Can you work these out from the model? Positions are in its coordinate system, mm. A direction names the side the tool comes from. Give positions to 0.01 mm unless a question says otherwise; leave off trailing zeros. Loops run counter-clockwise (first coordinate to the right, second up) from the corner with the lowest first, then second, coordinate; pieces in that order, holes last. Notation, with made-up numbers: (77, 85) - (131, 85) arc R13 cw to (131, 97) - close; hole circle Ø7 at (44.25, -14.5). An arc over 180 degrees is marked (long way). Answer as a JSON object with one key per item and string values.
```python
from build123d import *

# Parameters (mm, degrees)
SKETCH_1_W          = 68
SKETCH_1_H          = 65
EXTRUDE_1_DEPTH     = 68
SKETCH_2_W          = 65
SKETCH_2_H          = 65
CUT_EXTRUDE_1_DEPTH = 65
FILLET_1_R          = 1
SKETCH_6_R          = 2.6
SKETCH_6_R_2        = 19.1
CUT_EXTRUDE_4_DEPTH = 51
CUT_EXTRUDE_5_DEPTH = 51


with BuildPart() as part:
    # 草图1 → 凸台-拉伸1 (new body)
    with BuildSketch(Plane(origin=(0, 0, 0), x_dir=(0, 0, -1), z_dir=(1, 0, 0))):
        Rectangle(SKETCH_1_W, SKETCH_1_H)
    extrude(amount=EXTRUDE_1_DEPTH)

    # 草图2 → 切除-拉伸1 (cut)
    with BuildSketch(Plane(origin=(68, 0, 0), x_dir=(0, 0, -1), z_dir=(1, 0, 0))):
        with Locations((1.5, 0)):
            Rectangle(SKETCH_2_W, SKETCH_2_H)
    extrude(amount=-CUT_EXTRUDE_1_DEPTH, mode=Mode.SUBTRACT)

    # 圆角1
    fillet_1_edges = [part.edges().sort_by_distance(p)[0] for p in [
        (0, 0, 34),
    ]]
    fillet(fillet_1_edges, radius=FILLET_1_R)

    # 草图6 → 切除-拉伸4 (cut)
    with BuildSketch(Plane(origin=(0, 0, 31), x_dir=(-1, 0, 0), z_dir=(0, 0, -1))):
        with Locations((-62.5, 23.5)):
            Circle(SKETCH_6_R)
        with Locations((-15.5, 23.5)):
            Circle(SKETCH_6_R)
        with Locations((-39, 0)):
            Circle(SKETCH_6_R_2)
        with Locations((-15.5, -23.5)):
            Circle(SKETCH_6_R)
        with Locations((-62.5, -23.5)):
            Circle(SKETCH_6_R)
        Polygon((-68, 32.5), (-68, 27), (-62.5, 32.5), align=None)
        Polygon((-68, -27), (-62.5, -32.5), (-68, -32.5), align=None)
    extrude(amount=-CUT_EXTRUDE_4_DEPTH, mode=Mode.SUBTRACT)

    # 草图7 → 切除-拉伸5 (cut)
    with BuildSketch(Plane(origin=(3, 0, 0), x_dir=(0, 0, -1), z_dir=(1, 0, 0))):
        Polygon((28.5, 32.5), (34, 32.5), (34, 27), align=None)
        with BuildLine():
            Line((-18, 22.1), (24, 22.1))
            ThreePointArc((24, 22.1), (26.1, 20), (24, 17.9))
            Line((24, 17.9), (-18, 17.9))
            ThreePointArc((-18, 17.9), (-20.1, 20), (-18, 22.1))
        make_face()
        Polygon((34, -32.5), (34, -27), (28.5, -32.5), align=None)
        with BuildLine():
            Line((-18, -17.9), (24, -17.9))
            ThreePointArc((24, -17.9), (26.1, -20), (24, -22.1))
            Line((24, -22.1), (-18, -22.1))
            ThreePointArc((-18, -22.1), (-20.1, -20), (-18, -17.9))
        make_face()
    extrude(amount=-CUT_EXTRUDE_5_DEPTH, mode=Mode.SUBTRACT)


solid = part.part
```
1) Imagine slicing it at B-B on z = -18. Write out the boundary of the cut face in (x, y).
Check sheet entries:
{"outline": "(0, -32.5) - (3, -32.5) - (3, -22.1) - (0, -22.1) - close; (0, -17.9) - (3, -17.9) - (3, 17.9) - (0, 17.9) - close; (0, 22.1) - (3, 22.1) - (3, 32.5) - (0, 32.5) - close"}
2) Imagine slicing it at A-A on y = 23.5. Write out the boundary of the cut face in (x, z).
Check sheet entries:
{"outline": "(0, -34) - (3, -34) - (3, 31) - (12.9, 31) - (12.9, 34) - (1, 34) arc R1 ccw to (0, 33) - close; (18.1, 31) - (59.9, 31) - (59.9, 34) - (18.1, 34) - close; (65.1, 31) - (68, 31) - (68, 34) - (65.1, 34) - close"}
3) Which directions (+Z, -Z, +X, -X, +Y, -Y) give clear straight access to the entire face, cutting with the end or side of a thin tool? Please do faces 1 (the flat face through (65, 30, 32)), 2 (the cylindrical face through (1.5, 20, -26.1)), 3 (the flat face through (22, -15, 31)).
Check sheet entries:
{"face 1": "+Z, -Z, +X, +Y", "face 2": "+X, -X", "face 3": "-Z, +X, +Y, -Y"}
4) If we mould it in two halves opening along Y, with no side actions, what happens to faces 4 (the flat face through (19, 0, 34)), 5 (the cylindrical face through (14.1, 25.69, 32.48)), 6 (the flat face through (17, 32.5, 33))? For each: released by +Y, released by -Y, zero draft, split by the parting line, or undercut.
Check sheet entries:
{"face 4": "zero draft", "face 5": "undercut", "face 6": "released by +Y"}
5) I need wall thicknesses on L1, parallel to Y at x = 62.5, z = 32.05; L2, parallel to X at y = 28, z = -8; L3, parallel to Z at x = 60, y = 4.5. Which ranges of each line are inside material? Lowest first, please.
Check sheet entries:
{"L1": "-32.5 to -26.1, -20.9 to 20.9, 26.1 to 32.5", "L2": "0 to 3", "L3": "31 to 34"}
6) Imagine slicing it at C-C on x = 39. Write out the boundary of the cut face in (y, z), and give its area (3 significant figures).
Check sheet entries:
{"outline": "(-32.5, 31) - (-19.1, 31) - (-19.1, 34) - (-32.5, 34) - close; (19.1, 31) - (32.5, 31) - (32.5, 34) - (19.1, 34) - close", "area": "80.4 mm2"}
7) I'm going to push a flat-ended pin straight in: P1, Ø2, axis at y = 6, z = 18.5, coming from the +X side. Where does the tip first touch, or does it pass through?
Check sheet entries:
{"P1": "x = 3"}
8) Imagine slicing it at D-D on y = 15.5. Write out the boundary of the cut face in (x, z), and give its area (3 significant figures).
Check sheet entries:
{"outline": "(0, -34) - (3, -34) - (3, 31) - (27.84, 31) - (27.84, 34) - (1, 34) arc R1 ccw to (0, 33) - close; (50.16, 31) - (68, 31) - (68, 34) - (50.16, 34) - close", "area": "332 mm2"}
